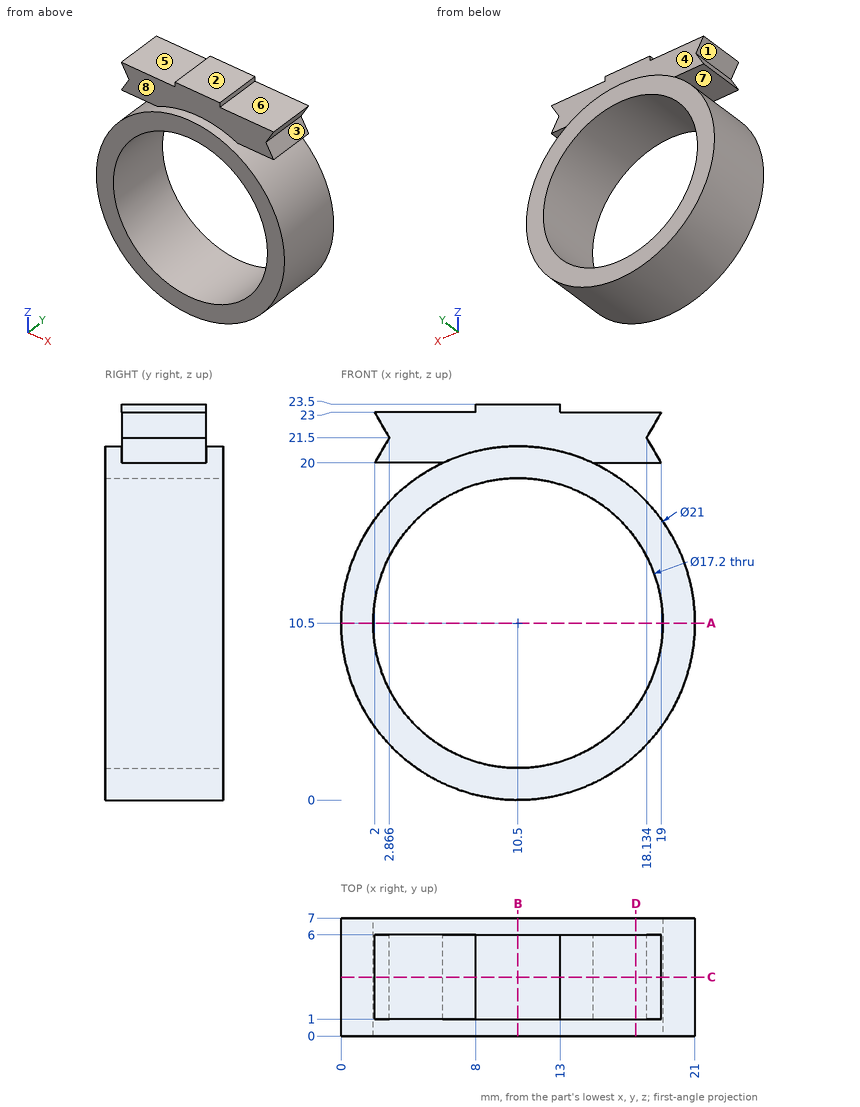
Design review of the part shown in the three views and the two pictorial views. Dimensions are in mm from the part's minimum x, y and z. A direction names the side the tool comes from. Give positions to 0.01 mm unless a question says otherwise; leave off trailing zeros. Loops run counter-clockwise (first coordinate to the right, second up) from the corner with the lowest first, then second, coordinate; pieces in that order, holes last. Notation, with made-up numbers: (14, 22.5) - (31, 22.5) arc R36 cw to (31, 61.5) - close; hole circle Ø6 at (37.25, 81). An arc over 180 degrees is marked (long way). Write item = value, one per line.
1) Take a section at D-D on x = 17.5. State the section outline as (y, z) points, and give its area (3 significant figures).
Result sheet:
outline = (0, 2.67) - (7, 2.67) - (7, 5.5) - (0, 5.5) - close; (0, 15.5) - (7, 15.5) - (7, 18.33) - (0, 18.33) - close; (1, 20) - (6, 20) - (6, 23) - (1, 23) - close
area = 54.6 mm2
2) Take a section at A-A on z = 10.5. State the section outline as (x, y) points.
Result sheet:
outline = (0, 0) - (1.9, 0) - (1.9, 7) - (0, 7) - close; (19.1, 0) - (21, 0) - (21, 7) - (19.1, 7) - close
3) Take a section at B-B on x = 10.5. State the section outline as (y, z) points.
Result sheet:
outline = (0, 0) - (7, 0) - (7, 1.9) - (0, 1.9) - close; (0, 19.1) - (7, 19.1) - (7, 21) - (6, 21) - (6, 23.5) - (1, 23.5) - (1, 21) - (0, 21) - close
4) Tool access review of the marked faces 1, 2, 3, 4 and 5: name each direction out of +Z, -Z, +X, -X, +Y, -Y from which nothing blocks a thin tool from reaching the whole face with its end or side.
Result sheet:
face_1 = -X, +Y, -Y
face_2 = +Z, +X, -X, +Y, -Y
face_3 = +X, +Y, -Y
face_4 = +Z, +Y
face_5 = +Z, -X, +Y, -Y
5) To check wall thickness, follow line 1 (Z direction, x = 10.5, y = 3.75); line 2 (X direction, y = 1.75, z = 10.5); line 3 (Z direction, x = 16, y = 5.5). State the ranges of each line that lie inside material, in increasing order.
Result sheet:
line_1 = 0 to 1.9, 19.1 to 23.5
line_2 = 0 to 1.9, 19.1 to 21
line_3 = 1.56 to 3.89, 17.11 to 19.44, 20 to 23
6) Draft analysis for pull direction Z (two halves, no side actions). For the marked faces 6, 7 and 8, state which applies: +Z half, -Z half, draft (parallel to the pull), parting line (faces both ways), or undercut.
Result sheet:
face_6 = +Z half
face_7 = undercut
face_8 = draft
7) Take a section at C-C on y = 3.5. State the section outline as (x, z) points, and give its area (3 significant figures).
Result sheet:
outline = (2, 20) - (6.03, 20) arc R10.5 ccw (long way) to (14.97, 20) - (19, 20) - (18.13, 21.5) - (19, 23) - (13, 23) - (13, 23.5) - (8, 23.5) - (8, 23) - (2, 23) - (2.87, 21.5) - close; hole circle Ø17.2 at (10.5, 10.5)
area = 159 mm2
8) Clearance check with flat-ended pins moving along their axes: pin 1 Ø3 at (y, z) = (3.5, 19) entering from -X; pin 2 Ø4 at (x, y) = (17, 4.5) entering from -Z; pin 3 Ø1.2 at (x, y) = (17.5, 2.5) entering from -Z. State where each tip first meets the part, or that it passes through.
Result sheet:
pin_1 = 2
pin_2 = 1.01
pin_3 = 2.18
